The model under review builds one solid part; all positions refer to its coordinate system, in mm. A direction names the side the tool comes from. Round coordinates to 2 decimals unless told otherwise and drop trailing zeros. Write each loop counter-clockwise with the first axis right and the second up, starting at its lowest first coordinate (ties: lowest second). Pieces come first, ordered by that corner, then holes. Notation, with made-up numbers: M -26.5,18.25 L -3.5,18.25 A31 cw -3.5,53.25 Z; hole C 59.5,-1 d4. An arc over 180 degrees is marked long. One line per item, written item: value. Start each with the question number.
1) Take a section at A-A, the plane x = 38.1. Write out the cut boundary in (y, z) (1 decimal).
2) Wall thickness on probe 1 along X at (y, z) = (3.5, -11.5) (1 decimal); probe 2 along X at (y, z) = (5.5, -24); probe 3 along Y at (x, z) = (8.5, -17.5): over which ranges is each line inside the solid? List them lowest first.
3) Tool access review of faces 4 (the face through (45, 3.969, -13)), 5 (the face through (3, 3.572, -13)), 6 (the face through (20.638, 4, -21)): name each direction out of +Z, -Z, +X, -X, +Y, -Y from which nothing blocks a thin tool from reaching the whole face with its end or side.
4) For P1, Ø2.5, axis at x = 9.5, z = -24, coming from the +Y side; P2, Ø1.3, axis at x = 38.1, z = -23.81, coming from the -Y side; P3, Ø0.5, axis at x = 48.5, y = 3.5, coming from the -Z side; P4, Ø15, axis at x = 52, z = -16, coming from the +Y side, all flat-tipped, find the tip position at first contact; note any pin that passes through.
5) Take a section at C-C, the plane z = -7.25. Write out the cut boundary in (x, y) (1 decimal), and give its area (3 significant figures).
6) Mouldability with a two-part tool opening along Z and no side actions: class faces 1 (the face through (45, 3, -4.762)), 2 (the face through (55.44, 0.8, -23.39)), 3 (the face through (60.325, 1, -13)) as +Z half, -Z half, draft (parallel to the pull), parting line (faces both ways), or undercut.
7) Take a section at B-B, the plane x = 19.05. Write out the cut boundary in (y, z), and give its area (3 significant figures).
8) Take a section at D-D, the plane z = -16.5. Write out the cut boundary in (x, y) (1 decimal), and give its area (3 significant figures).
from build123d import *

# Parameters (mm, degrees)
BOSS_EXTRUDE1_DEPTH = 1.5875
SKETCH2_W           = 7.9375
SKETCH2_H           = 9.525
BOSS_EXTRUDE2_DEPTH = 3.175
CUT_EXTRUDE2_DEPTH  = 7.9375
SKETCH4_W           = 6.35
SKETCH4_H           = 0.79375
CUT_EXTRUDE3_DEPTH  = 5.3975
SKETCH5_W           = 1.5875
SKETCH5_H           = 9.525
CUT_EXTRUDE4_DEPTH  = 1.5875
SKETCH6_R           = 1.27
CUT_EXTRUDE5_DEPTH  = 1.5875
SKETCH7_W           = 25.4
SKETCH7_H           = 19.05
SKETCH7_W_2         = 17.62125
SKETCH7_H_2         = 15.875
SKETCH7_W_3         = 4.7625
SKETCH7_H_3         = 3.175
SKETCH7_W_4         = 7.9375
SKETCH7_H_4         = 7.9375
SKETCH7_W_5         = 2.38125
SKETCH7_H_5         = 12.7
BOSS_EXTRUDE3_DEPTH = 3.175
SKETCH10_W          = 7.9375
SKETCH10_H          = 7.9375
BOSS_EXTRUDE4_DEPTH = 2.38125
SKETCH11_W          = 2.38125
SKETCH11_H          = 12.7
BOSS_EXTRUDE5_DEPTH = 0.79375
SKETCH12_W          = 25.4
SKETCH12_H          = 19.05
CUT_EXTRUDE6_DEPTH  = 0.79375
SKETCH13_W          = 25.4
SKETCH13_H          = 19.05
SKETCH13_W_2        = 17.4625
SKETCH13_H_2        = 15.875
CUT_EXTRUDE7_DEPTH  = 1.5875
SKETCH14_R          = 0.79375
CUT_EXTRUDE8_DEPTH  = 1.5875


with BuildPart() as part:
    # Sketch1 → Boss-Extrude1 (new body)
    with BuildSketch(Plane(origin=(0, 0, 0), x_dir=(1, 0, 0), z_dir=(0, 1, 0))):
        Polygon((1.5875, 7.9375), (1.5875, 0), (60.325, 0), (60.325, 25.4), (1.5875, 25.4), (1.5875, 17.4625), (0, 17.4625), (0, 7.9375), align=None)
    extrude(amount=BOSS_EXTRUDE1_DEPTH)

    # Sketch2 → Boss-Extrude2 (add)
    with BuildSketch(Plane(origin=(0, 1.5875, 0), x_dir=(1, 0, 0), z_dir=(0, 1, 0))):
        with Locations((3.96875, 12.7)):
            Rectangle(SKETCH2_W, SKETCH2_H)
    extrude(amount=BOSS_EXTRUDE2_DEPTH)

    # Sketch3 → Cut-Extrude2 (cut)
    with BuildSketch(Plane.ZY):
        with BuildLine():
            Line((-15.875, 4.7625), (-17.4625, 4.7625))
            Line((-17.4625, 4.7625), (-17.4625, 3.175))
            ThreePointArc((-17.4625, 3.175), (-16.997532015, 4.297532015), (-15.875, 4.7625))
        make_face()
        with BuildLine():
            ThreePointArc((-15.875, 1.5875), (-16.997532015, 2.052467985), (-17.4625, 3.175))
            Line((-17.4625, 3.175), (-17.4625, 1.5875))
            Line((-17.4625, 1.5875), (-15.875, 1.5875))
        make_face()
        with BuildLine():
            Line((-7.9375, 4.7625), (-9.525, 4.7625))
            ThreePointArc((-9.525, 4.7625), (-8.402467985, 4.297532015), (-7.9375, 3.175))
            Line((-7.9375, 3.175), (-7.9375, 4.7625))
        make_face()
        with BuildLine():
            Line((-7.9375, 1.5875), (-7.9375, 3.175))
            ThreePointArc((-7.9375, 3.175), (-8.402467985, 2.052467985), (-9.525, 1.5875))
            Line((-9.525, 1.5875), (-7.9375, 1.5875))
        make_face()
    extrude(amount=-CUT_EXTRUDE2_DEPTH, mode=Mode.SUBTRACT)

    # Sketch4 → Cut-Extrude3 (cut)
    with BuildSketch(Plane.ZY):
        with BuildLine():
            Line((-15.875, 1.984375), (-9.525, 1.984375))
            ThreePointArc((-9.525, 1.984375), (-8.334375, 3.175), (-9.525, 4.365625))
            Line((-9.525, 4.365625), (-15.875, 4.365625))
            ThreePointArc((-15.875, 4.365625), (-17.065625, 3.175), (-15.875, 1.984375))
        make_face()
        with Locations((-12.7, 3.175)):
            Rectangle(SKETCH4_W, SKETCH4_H, mode=Mode.SUBTRACT)
    extrude(amount=-CUT_EXTRUDE3_DEPTH, mode=Mode.SUBTRACT)

    # Sketch5 → Cut-Extrude4 (cut)
    with BuildSketch(Plane.XZ):
        with Locations((0.79375, -12.7)):
            Rectangle(SKETCH5_W, SKETCH5_H)
    extrude(amount=-CUT_EXTRUDE4_DEPTH, mode=Mode.SUBTRACT)

    # Sketch6 → Cut-Extrude5 (cut)
    with BuildSketch(Plane(origin=(0, 1.5875, 0), x_dir=(1, 0, 0), z_dir=(0, 1, 0))):
        with BuildLine():
            ThreePointArc((1.5875, 24.13), (1.959474388, 25.028025612), (2.8575, 25.4))
            Line((2.8575, 25.4), (1.5875, 25.4))
            Line((1.5875, 25.4), (1.5875, 24.13))
        make_face()
        with BuildLine():
            ThreePointArc((2.8575, 0), (1.959474388, 0.371974388), (1.5875, 1.27))
            Line((1.5875, 1.27), (1.5875, 0))
            Line((1.5875, 0), (2.8575, 0))
        make_face()
        with BuildLine():
            Line((60.325, 0), (60.325, 1.27))
            ThreePointArc((60.325, 1.27), (59.953025612, 0.371974388), (59.055, 0))
            Line((59.055, 0), (60.325, 0))
        make_face()
        with BuildLine():
            Line((60.325, 25.4), (59.055, 25.4))
            ThreePointArc((59.055, 25.4), (59.953025612, 25.028025612), (60.325, 24.13))
            Line((60.325, 24.13), (60.325, 25.4))
        make_face()
        with Locations(Location((3.175, 23.8125, 0), (0, 0, 270))):
            Circle(SKETCH6_R)
        with Locations(Location((3.175, 1.5875, 0), (0, 0, 270))):
            Circle(SKETCH6_R)
        with Locations(Location((58.7375, 1.5875, 0), (0, 0, 270))):
            Circle(SKETCH6_R)
        with Locations(Location((58.7375, 23.8125, 0), (0, 0, 270))):
            Circle(SKETCH6_R)
    extrude(amount=-CUT_EXTRUDE5_DEPTH, mode=Mode.SUBTRACT)

    # Sketch7 → Boss-Extrude3 (add)
    with BuildSketch(Plane(origin=(0, 1.5875, 0), x_dir=(1, 0, 0), z_dir=(0, 1, 0))):
        with Locations((47.625, 12.7)):
            Rectangle(SKETCH7_W, SKETCH7_H)
        with Locations((45.323125, 12.7)):
            Rectangle(SKETCH7_W_2, SKETCH7_H_2, mode=Mode.SUBTRACT)
        with Locations((45.323125, 12.7)):
            Rectangle(SKETCH7_W_2, SKETCH7_H_2)
        with Locations((8.73125, 23.8125)):
            Rectangle(SKETCH7_W_3, SKETCH7_H_3)
        with Locations((8.73125, 1.5875)):
            Rectangle(SKETCH7_W_3, SKETCH7_H_3)
        with Locations((16.66875, 21.43125)):
            Rectangle(SKETCH7_W_4, SKETCH7_H_4)
        with Locations((31.353125, 12.7)):
            Rectangle(SKETCH7_W_5, SKETCH7_H_5)
    extrude(amount=BOSS_EXTRUDE3_DEPTH)

    # Sketch10 → Boss-Extrude4 (add)
    with BuildSketch(Plane(origin=(0, 4.7625, 0), x_dir=(1, 0, 0), z_dir=(0, 1, 0))):
        with Locations((16.66875, 21.43125)):
            Rectangle(SKETCH10_W, SKETCH10_H)
    extrude(amount=BOSS_EXTRUDE4_DEPTH)

    # Sketch11 → Boss-Extrude5 (add)
    with BuildSketch(Plane(origin=(0, 4.7625, 0), x_dir=(1, 0, 0), z_dir=(0, 1, 0))):
        with Locations((31.353125, 12.7)):
            Rectangle(SKETCH11_W, SKETCH11_H)
    extrude(amount=BOSS_EXTRUDE5_DEPTH)

    # Sketch12 → Cut-Extrude6 (cut)
    with BuildSketch(Plane(origin=(0, 4.7625, 0), x_dir=(1, 0, 0), z_dir=(0, 1, 0))):
        with Locations((47.625, 12.7)):
            Rectangle(SKETCH12_W, SKETCH12_H)
    extrude(amount=-CUT_EXTRUDE6_DEPTH, mode=Mode.SUBTRACT)

    # Sketch13 → Cut-Extrude7 (cut)
    with BuildSketch(Plane(origin=(0, 3.96875, 0), x_dir=(1, 0, 0), z_dir=(0, 1, 0))):
        with Locations((47.625, 12.7)):
            Rectangle(SKETCH13_W, SKETCH13_H)
        with Locations((45.24375, 12.7)):
            Rectangle(SKETCH13_W_2, SKETCH13_H_2, mode=Mode.SUBTRACT)
    extrude(amount=-CUT_EXTRUDE7_DEPTH, mode=Mode.SUBTRACT)

    # Sketch14 → Cut-Extrude8 (cut)
    with BuildSketch(Plane(origin=(0, 1.5875, 0), x_dir=(1, 0, 0), z_dir=(0, 1, 0))):
        with Locations(Location((23.8125, 23.8125, 0), (0, 0, 270))):
            Circle(SKETCH14_R)
        with Locations(Location((26.19375, 23.8125, 0), (0, 0, 270))):
            Circle(SKETCH14_R)
        with Locations(Location((28.575, 23.8125, 0), (0, 0, 270))):
            Circle(SKETCH14_R)
        with Locations(Location((30.95625, 23.8125, 0), (0, 0, 270))):
            Circle(SKETCH14_R)
        with Locations(Location((38.1, 23.8125, 0), (0, 0, 270))):
            Circle(SKETCH14_R)
        with Locations(Location((42.8625, 23.8125, 0), (0, 0, 270))):
            Circle(SKETCH14_R)
        with Locations(Location((33.3375, 23.8125, 0), (0, 0, 270))):
            Circle(SKETCH14_R)
        with Locations(Location((35.71875, 23.8125, 0), (0, 0, 270))):
            Circle(SKETCH14_R)
        with Locations(Location((40.48125, 23.8125, 0), (0, 0, 270))):
            Circle(SKETCH14_R)
        with Locations(Location((45.24375, 23.8125, 0), (0, 0, 270))):
            Circle(SKETCH14_R)
        with Locations(Location((47.625, 23.8125, 0), (0, 0, 270))):
            Circle(SKETCH14_R)
        with Locations(Location((50.00625, 23.8125, 0), (0, 0, 270))):
            Circle(SKETCH14_R)
        with Locations(Location((52.3875, 23.8125, 0), (0, 0, 270))):
            Circle(SKETCH14_R)
        with Locations(Location((54.76875, 23.8125, 0), (0, 0, 270))):
            Circle(SKETCH14_R)
        with Locations(Location((14.2875, 1.5875, 0), (0, 0, 270))):
            Circle(SKETCH14_R)
        with Locations(Location((16.66875, 1.5875, 0), (0, 0, 270))):
            Circle(SKETCH14_R)
        with Locations(Location((19.05, 1.5875, 0), (0, 0, 270))):
            Circle(SKETCH14_R)
        with Locations(Location((21.43125, 1.5875, 0), (0, 0, 270))):
            Circle(SKETCH14_R)
        with Locations(Location((23.8125, 1.5875, 0), (0, 0, 270))):
            Circle(SKETCH14_R)
        with Locations(Location((26.19375, 1.5875, 0), (0, 0, 270))):
            Circle(SKETCH14_R)
        with Locations(Location((28.575, 1.5875, 0), (0, 0, 270))):
            Circle(SKETCH14_R)
        with Locations(Location((30.95625, 1.5875, 0), (0, 0, 270))):
            Circle(SKETCH14_R)
        with Locations(Location((33.3375, 1.5875, 0), (0, 0, 270))):
            Circle(SKETCH14_R)
        with Locations(Location((35.71875, 1.5875, 0), (0, 0, 270))):
            Circle(SKETCH14_R)
        with Locations(Location((38.1, 1.5875, 0), (0, 0, 270))):
            Circle(SKETCH14_R)
        with Locations(Location((40.48125, 1.5875, 0), (0, 0, 270))):
            Circle(SKETCH14_R)
        with Locations(Location((42.8625, 1.5875, 0), (0, 0, 270))):
            Circle(SKETCH14_R)
        with Locations(Location((45.24375, 1.5875, 0), (0, 0, 270))):
            Circle(SKETCH14_R)
        with Locations(Location((47.625, 1.5875, 0), (0, 0, 270))):
            Circle(SKETCH14_R)
        with Locations(Location((50.00625, 1.5875, 0), (0, 0, 270))):
            Circle(SKETCH14_R)
        with Locations(Location((52.3875, 1.5875, 0), (0, 0, 270))):
            Circle(SKETCH14_R)
        with Locations(Location((54.76875, 1.5875, 0), (0, 0, 270))):
            Circle(SKETCH14_R)
    extrude(amount=-CUT_EXTRUDE8_DEPTH, mode=Mode.SUBTRACT)


solid = part.part
Checked values:
1. outline: M 0,-25.4 L 1.6,-25.4 L 1.6,-24.6 L 0,-24.6 Z; M 0,-23 L 1.6,-23 L 1.6,-22.2 L 2.4,-22.2 L 2.4,-20.6 L 4,-20.6 L 4,-4.8 L 2.4,-4.8 L 2.4,-3.2 L 1.6,-3.2 L 1.6,-2.4 L 0,-2.4 Z; M 0,-0.8 L 1.6,-0.8 L 1.6,0 L 0,0 Z
2. probe 1: x = 0 to 7.9, 30.2 to 32.5, 36.5 to 54
2. probe 2: x = 12.7 to 20.64
2. probe 3: y = 0 to 1.59
3. face 4: +Z, -Z, +X, +Y
3. face 5: -X
3. face 6: +Z, -Z, +Y
4. P1: stops at y = 4.76
4. P2: passes through
4. P3: stops at z = -20.64
4. P4: stops at y = 3.97
5. outline: M 1.6,0 L 60.3,0 L 60.3,2.4 L 54,2.4 L 54,4 L 36.5,4 L 36.5,2.4 L 34.9,2.4 L 34.9,1.6 L 32.5,1.6 L 32.5,5.6 L 30.2,5.6 L 30.2,1.6 L 1.6,1.6 Z
5. area: 151 mm2
6. face 1: +Z half
6. face 2: undercut
6. face 3: draft
7. outline: M 0,-25.4 L 7.14,-25.4 L 7.14,-17.46 L 1.59,-17.46 L 1.59,-2.38 L 0,-2.38 Z; M 0,-0.79 L 1.59,-0.79 L 1.59,0 L 0,0 Z
7. area: 81.9 mm2
8. outline: M 0,1.7 L 7.9,1.7 L 7.9,4.6 L 0,4.6 L 0,4.2 L 5.4,4.2 L 5.4,2.2 L 0,2.2 Z; M 1.6,0 L 60.3,0 L 60.3,2.4 L 54,2.4 L 54,4 L 36.5,4 L 36.5,2.4 L 34.9,2.4 L 34.9,1.6 L 32.5,1.6 L 32.5,5.6 L 30.2,5.6 L 30.2,1.6 L 1.6,1.6 Z
8. area: 163 mm2
